Build history of the part. All positions in model axes, mm. A direction names the side the tool comes from. Round coordinates to 2 decimals unless told otherwise and drop trailing zeros. Loops run counter-clockwise (first coordinate to the right, second up) from the corner with the lowest first, then second, coordinate; pieces in that order, holes last. Notation, with made-up numbers: (-28, 34.25) -> (24, 34.25) arc R18 cw to (24, 59.25) -> close; hole circle Ø3 at (10.25, 43). An arc over 180 degrees is marked (long way). Put each result on its own line as item: value. Start each with the question number.
Item 1: Cut at D-D, the plane y = -18. List the corners of the cut face in (x, z), plus the area to 3 significant figures.
Item 2: Pull direction X, two halves, no side cores. Call faces 1 (the flat face through (0, 11, -8)), 2 (the flat face through (24.638, 21, 11)), 3 (the flat face through (44, 2, -27.631)): +X half, -X half, draft (parallel to the pull), parting line (faces both ways), or undercut.
Item 3: Drill centre lines: probe 1 along X at (y, z) = (15, 0); probe 2 along Z at (x, y) = (76.5, -21); probe 3 along Y at (x, z) = (13.5, 5.5). Where is each one in solid material? Low to high. Write a range as [from, to].
Item 4: Cut at A-A, the plane z = 16.5. List the corners of the cut face in (x, y), plus the area to 3 significant figures.
Item 5: Cut at C-C, the plane x = 10. List the corners of the cut face in (y, z), plus the area to 3 significant figures.
Item 6: Tool access for faces 4 (the flat face through (76, 2.567, 11)), 5 (the flat face through (64.012, 21, 10)), 6 (the flat face through (44, 40.667, -8)): list every direction of +Z, -Z, +X, -X, +Y, -Y with a clear straight run to the whole face (end or side of a thin tool).
Item 7: Flat gauge pins, fed straight in: pin 1 Ø19.5 at (x, z) = (10.5, 5) entering from -Y; pin 2 Ø12.5 at (x, z) = (72.5, 14) entering from -Y. Where does each tip first touch, or does it go through?
Item 8: Cut at B-B, the plane y = 18. List the corners of the cut face in (x, z).
```python
from build123d import *

# Parameters (mm, degrees)
F1_DEPTH  = 88.9
F2_W      = 19.562296
F2_H      = 25.4
F3_DEPTH  = 38.101
F3_FACE_W = 38.1
F3_FACE_H = 25.4
F4_DEPTH  = 19.812


with BuildPart() as f1:
    # F0 (on Right) → F1 (new body)
    with BuildSketch(Plane.YZ):
        Polygon((-35.532832, -2.230505), (-35.532832, -27.630505), (40.667168, -27.630505), (40.667168, 23.169495), (2.567168, 23.169495), (2.567168, -2.230505), align=None)
    extrude(amount=F1_DEPTH)

    # F2 (on face) → F3 (cut, through all)
    with BuildSketch(Plane.XZ.offset(-2.567168)):
        with Locations((54.231148, 10.469495)):
            Rectangle(F2_W, F2_H)
    extrude(amount=-F3_DEPTH, mode=Mode.SUBTRACT)

    # F3_face (on face) → F4 (cut)
    with BuildSketch(Plane(origin=(44.45, 21.617168, 10.469495), x_dir=(0, 1, 0), z_dir=(1, 0, 0))):
        Rectangle(F3_FACE_W, F3_FACE_H)
    extrude(amount=-F4_DEPTH, mode=Mode.SUBTRACT)


solid = f1.part
```
Reply:
1. outline: (0, -27.63) -> (88.9, -27.63) -> (88.9, -2.23) -> (0, -2.23) -> close
1. area: 2,260 mm^2
2. face 1: -X half
2. face 2: undercut
2. face 3: draft
3. probe 1: x = [0, 24.64], [64.01, 88.9]
3. probe 2: z = [-27.63, -2.23]
3. probe 3: y = [2.57, 40.67]
4. outline: (0, 2.57) -> (24.64, 2.57) -> (24.64, 40.67) -> (0, 40.67) -> close; (64.01, 2.57) -> (88.9, 2.57) -> (88.9, 40.67) -> (64.01, 40.67) -> close
4. area: 1,890 mm^2
5. outline: (-35.53, -27.63) -> (40.67, -27.63) -> (40.67, 23.17) -> (2.57, 23.17) -> (2.57, -2.23) -> (-35.53, -2.23) -> close
5. area: 2,900 mm^2
6. face 4: +Z, +X, -X, -Y
6. face 5: +Z, +Y, -Y
6. face 6: +Z, -Z, +X, -X, +Y
7. pin 1: stops at y = -35.53
7. pin 2: stops at y = 2.57
8. outline: (0, -27.63) -> (88.9, -27.63) -> (88.9, 23.17) -> (64.01, 23.17) -> (64.01, -2.23) -> (24.64, -2.23) -> (24.64, 23.17) -> (0, 23.17) -> close
